Input: part model. Units: mm. Frame: model coordinates. Round coordinates to 2 decimals unless told otherwise and drop trailing zeros. Order: outer loops, then holes, each group sorted by start corner. A loop starts at its lowest first (then second) coordinate and runs counter-clockwise, first axis right, second up.
Item 1: Cut plane A-A on z = 0. Output: boundary loops of the cut face in (x, y), then the cut area to 3 significant figures.
Item 2: Line query: L1, parallel to Z at x = 5.5, y = -0.25; L2, parallel to Y at x = 104, z = -0.5; L3, parallel to Z at x = 61.5, y = 5. Output: solid intervals per line, ascending.
Item 3: First-contact query: pin 1 (2 mm diameter, centred on x = 19.5, z = 5, fed in from +Y); pin 2 (1.2 mm diameter, centred on x = 5.5, y = 6.5, fed in from +Z); pin 3 (3 mm diameter, centred on x = 103, y = 5.5, fed in from -Z). Flat tips, straight axial feed; report the tip coordinate or a pass-through.
Item 4: Cut plane C-C on y = -2.25. Output: boundary loops of the cut face in (x, z), then the cut area to 3 significant figures.
Item 5: Cut plane B-B on x = 84. Output: boundary loops of the cut face in (y, z).
```python
from build123d import *

# Parameters (mm, degrees)
SKETCH1_R           = 7.5
BOSS_EXTRUDE1_DEPTH = 115
CUT_EXTRUDE3_START  = 10
CUT_EXTRUDE3_DEPTH  = 12.5
CUT_EXTRUDE4_START  = 10
CUT_EXTRUDE4_DEPTH  = 12.7


with BuildPart() as part:
    # Sketch1 → Boss-Extrude1 (new body)
    with BuildSketch(Plane(origin=(0, 0, 0), x_dir=(0, 0, -1), z_dir=(1, 0, 0))):
        Circle(SKETCH1_R)
    extrude(amount=BOSS_EXTRUDE1_DEPTH)

    # Sketch8 → Cut-Extrude3 (cut)
    with BuildSketch(Plane(origin=(0, 7.071067812, 0), x_dir=(1, 0, 0), z_dir=(0, 1, 0)).offset(CUT_EXTRUDE3_START)):
        with BuildLine():
            Line((0, 2.5), (17.5, 2.5))
            ThreePointArc((17.5, 2.5), (20, 0), (17.5, -2.5))
            Line((17.5, -2.5), (0, -2.5))
            ThreePointArc((0, -2.5), (-2.5, 0), (0, 2.5))
        make_face()
    extrude(amount=-CUT_EXTRUDE3_DEPTH, mode=Mode.SUBTRACT)

    # Sketch9 → Cut-Extrude4 (cut)
    with BuildSketch(Plane(origin=(0, 7.071067812, 0), x_dir=(1, 0, 0), z_dir=(0, 1, 0)).offset(CUT_EXTRUDE4_START)):
        with BuildLine():
            Line((115, -2.5), (97.5, -2.5))
            ThreePointArc((97.5, -2.5), (95, 0), (97.5, 2.5))
            Line((97.5, 2.5), (115, 2.5))
            ThreePointArc((115, 2.5), (117.5, 0), (115, -2.5))
        make_face()
    extrude(amount=-CUT_EXTRUDE4_DEPTH, mode=Mode.SUBTRACT)


solid = part.part
```
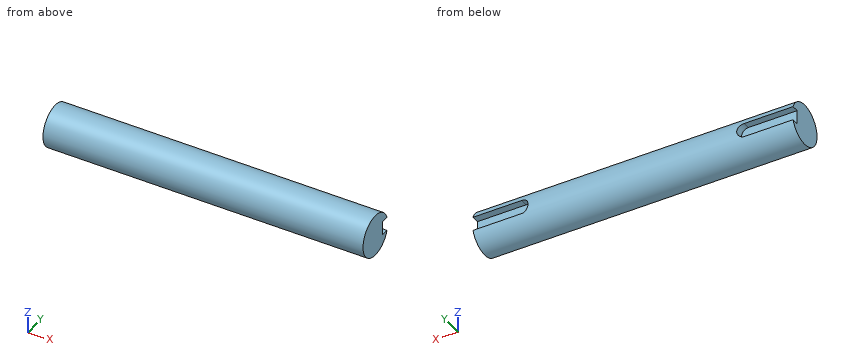
From the geometry:
1. outline: (0, -7.5) - (115, -7.5) - (115, 4.37) - (95, 4.37) - (95, 7.5) - (20, 7.5) - (20, 4.57) - (0, 4.57) - close
1. area: 1,600 mm2
2. L1: z = -7.5 to 7.5
2. L2: y = -7.48 to 4.37
2. L3: z = -5.59 to 5.59
3. pin 1: stops at y = 6.34
3. pin 2: stops at z = 4.63
3. pin 3: stops at z = -6.34
4. outline: (0, -7.15) - (115, -7.15) - (115, 7.15) - (0, 7.15) - close
4. area: 1,650 mm2
5. outline: circle Ø15 at (0, 0)
